Autodesk Inventor part; units mm, degrees
ref_plane "YZ Plane" through (0, 0, 0) normal (1, 0, 0) x (0, 1, 0)
ref_plane "XZ Plane" through (0, 0, 0) normal (0, 1, 0) x (-1, 0, 0)
ref_plane "XY Plane" through (0, 0, 0) normal (0, 0, 1) x (1, 0, 0)
sketch "スケッチ1" plane through (0, 0, 0) normal (0, 0, 1) x (1, 0, 0)
  circle A0 centre (0, 0) radius 6.25
  line L0 (0, 13) -> (-16, 13)
  line L1 (-16, 13) -> (-16, -13)
  line L2 (-16, -13) -> (0, -13)
  line L3 (0, -13) -> (0, 13)
  line L4 (0, 13) -> (3, 13)
  line L5 (3, 13) -> (3, -13)
  line L6 (3, -13) -> (0, -13)
  line L7 (0, -13) -> (0, 13)
  point P0 (-16, 0)
  point P1 (3, -5.4829)
  point P2 (3, 5.4829)
  dimension "d0" = 12.5
  dimension "d1" = 16
  dimension "d2" = 26
  dimension "d3" = 3
extrude "プレート1" add sketch "スケッチ1" along normal blind 1.5 contours A0 L3 L4 L5 | L5 L6 L3 A0 | A0 L3 L2 L1 L0
sketch "スケッチ2" plane through (-14.5, 13, 1.5) normal (-1, 0, 0) x (0, -1, 0)
  line L0 (26, 0) -> (0, 0)
  line L1 (0, 0) -> (0, -11)
  line L2 (0, -11) -> (26, -11)
  line L3 (26, -11) -> (26, 0)
edge flange "フランジ1" height 11 angle 90 thickness 1.5 bend radius 1.5 thickness toward (-1, 0, 0) relief tear relief width 1.5 relief depth 0.75 edges at (-16, 0, 0) wall of the first edge with corners at (-14.5, -13, 1.5) (-14.5, 13, 1.5) (-14.5, 13, -9.5) (-14.5, -13, -9.5)
bend "曲げ1"
corner "コーナー1"
sketch "スケッチ3" plane through (-16, -13, -9.5) normal (-1, 0, 0) x (0, 0, 1)
  line L0 (8, 0) -> (0, 0)
  line L1 (0, 0) -> (8, 0)
  line L2 (8, 0) -> (8, -26)
  line L3 (8, -26) -> (0, -26)
  line L4 (0, -26) -> (0, 0)
  line L5 (8, 0) -> (8, 26)
  arc A0 (0, 0) -> (3, 26) centre (-111.1667, 26) ccw
  line L6 (3, 20) -> (3, 26) construction
  line L7 (0, 26) -> (8, 26)
  line L8 (0, 0) -> (0, 26)
  point P0 (9.5, 13)
  point P1 (8, 0)
  dimension "d15" = 26
  dimension "d21" = 5
sheet face with bend "面2" sketch "スケッチ3" thickness 1.5 toward (1, 0, 0) bend radius 1.5 contours L2 L3 L4 L0
bend "曲げ2"
extrude "切り取り1" cut sketch "スケッチ3" against normal blind 1.5 contours L8 L7 A0
sketch "スケッチ5" plane through (0, 0, 0) normal (0, 0, -1) x (-1, 0, 0)
  circle A0 centre (0, 10.5) radius 0.85
  circle A1 centre (0, -10.5) radius 0.85
  point P0 (0, 0)
extrude "切り取り2" cut sketch "スケッチ5" against normal blind 1.5
sketch "スケッチ6" plane through (-16, -39, -1.5) normal (-1, 0, 0) x (0, 0, 1)
  circle A0 centre (-5, 23.5) radius 0.85
  circle A1 centre (-5, 2.5) radius 0.85
  point P0 (1.5, 39)
extrude "切り取り3" cut sketch "スケッチ6" against normal blind 1.5
fillet "フィレット1" radius 3 8 edges at (3, 13, 0.75) (3, 5.4829, 0.75) (3, -5.4829, 0.75) (3, -13, 0.75) (-15.25, -13, -9.5) (-15.25, 13, -6.5) (-15.25, -39, -9.5) (-15.25, -39, -1.5)
equation "\"d23\" = Thickness"
equation "\"d25\" = Thickness"
equation "\"d27\" = Thickness"
equation "\"d4\" = Thickness"
equation "\"d5\" = BendReliefWidth"
equation "\"d6\" = BendReliefDepth"
equation "\"d7\" = MinimumRemnant"
equation "\"d8\" = TransitionRadius"
equation "\"d11\" = BendRadius"
equation "\"d12\" = CornerReliefSize"
equation "\"d13\" = GapSize"
equation "\"d14\" = JacobiRadiusSize"
equation "\"d16\" = BendRadius"
equation "\"d17\" = BendReliefWidth"
equation "\"d19\" = MinimumRemnant"
equation "\"d18\" = BendReliefDepth"
equation "\"d20\" = TransitionRadius"
equation "\"BendRadius\" = Thickness"
equation "\"BendReliefWidth\" = Thickness"
equation "\"BendReliefDepth\" = 0.5 * Thickness"
equation "\"CornerReliefSize\" = 4 * Thickness"
equation "\"MinimumRemnant\" = 2 * Thickness"
equation "\"TransitionRadius\" = BendRadius"
equation "\"JacobiRadiusSize\" = BendRadius"
equation "\"GapSize\" = Thickness"
properties part number "hipjoint_toleg_under_right"
Work out the finished part from the listing and answer in its coordinate system (mm). A direction names the side the tool comes from. Give positions to 0.01 mm unless a question says otherwise; leave off trailing zeros. Order: outer loops, then holes, each group sorted by start corner. A loop starts at its lowest first (then second) coordinate and runs counter-clockwise, first axis right, second up. Notation, with made-up numbers: (17, 21) - (76, 21) arc R11 cw to (76, 29) - close; hole circle Ø10 at (19.5, 86). An arc over 180 degrees is marked (long way). Answer as CSV lines item,"result". Start each with the question number.
Q1. The part is cut by section B-B (x = -15). Write down the section's boundary in (y, z).
Q2. The part is cut by section C-C (z = 0.75). Write down the section's boundary in (x, y).
Q3. The part is cut by section D-D (y = -36.5). Write down the section's boundary in (x, z).
Q4. The part is cut by section A-A (y = -15.5). Write down the section's boundary in (x, z).
Q5. Find the intervals of material crossed by L1, parallel to Y at x = 0, z = 0.4; L2, parallel to X at y = 8.5, z = -6.25; L3, parallel to Z at x = -9, y = 9, in increasing order. Write a range as [from, to].
Q6. For faces 1 (the face through (-15, -24, -1.5)), 2 (the face through (2.1, 7.11, 0.76)), 3 (the face through (0.111, 11.343, 0.74)), determine the directions among +Z, -Z, +X, -X, +Y, -Y from which every point of the face is accessible in a straight line to the end or side of a thin tool.
Q7. The mould has two halves that part along Y. Classify faces 4 (the face through (2.14, -7.15, 0.76)), 5 (the face through (-7, 0, 0)), 6 (the face through (-15.26, -1.53, -7.43)): +Y half, -Y half, draft (parallel to the pull), parting line (faces both ways), or undercut.
Q8. Given pin 1 Ø1 at (y, z) = (-13, -6.5) entering from +X; pin 2 Ø6 at (x, z) = (-5, -5) entering from -Y; pin 3 Ø2 at (y, z) = (7.5, 0.5) entering from +X; pin 4 Ø2.5 at (x, z) = (-10, -0.5) entering from -Y, each flat-ended and moving along its own axis, determine where each tip first touches the part or whether it passes through.
Check result:
1,outline,"(-39, -6.5) arc R3 ccw to (-36, -9.5) - (-13.34, -9.5) arc R3 ccw to (-12.67, -9.42) arc R114.17 cw to (10.08, -6.54) arc R3 ccw to (13, -3.54) - (13, 0.74) - (-13, 0.74) - (-13, -1.5) - (-36, -1.5) arc R3 ccw to (-39, -4.5) - close; hole circle Ø1.7 at (-36.5, -6.5); hole circle Ø1.7 at (-15.5, -6.5)"
2,outline,"(-14.98, -13) - (0, -13) arc R3 ccw to (3, -10) - (3, -9.25) arc R3 ccw to (0, -6.25) arc R6.25 cw to (0, 6.25) arc R3 ccw to (3, 9.25) - (3, 10) arc R3 ccw to (0, 13) - (-14.98, 13) - close; hole circle Ø1.7 at (0, -10.5); hole circle Ø1.7 at (0, 10.5)"
3,outline,"(-16, -9.46) - (-14.5, -9.46) - (-14.5, -7.35) - (-16, -7.35) - close; (-16, -5.65) - (-14.5, -5.65) - (-14.5, -1.54) - (-16, -1.54) - close"
4,outline,"(-16, -9.5) - (-14.5, -9.5) - (-14.5, -7.35) - (-16, -7.35) - close; (-16, -5.65) - (-14.5, -5.65) - (-14.5, -1.5) - (-16, -1.5) - close"
5,L1,"y = [-13, -11.35], [-9.65, -6.25], [6.25, 9.65], [11.35, 13]"
5,L2,"x = [-16, -14.5]"
5,L3,"z = [0, 1.5]"
6,face 1,"+Z, +X, -X, -Y"
6,face 2,"+Z, -Z, +X"
6,face 3,"+Z, -Z"
7,face 4,"undercut"
7,face 5,"draft"
7,face 6,"+Y half"
8,pin 1,"stops at x = -14.5"
8,pin 2,"passes through"
8,pin 3,"stops at x = 2.9"
8,pin 4,"stops at y = -13"
